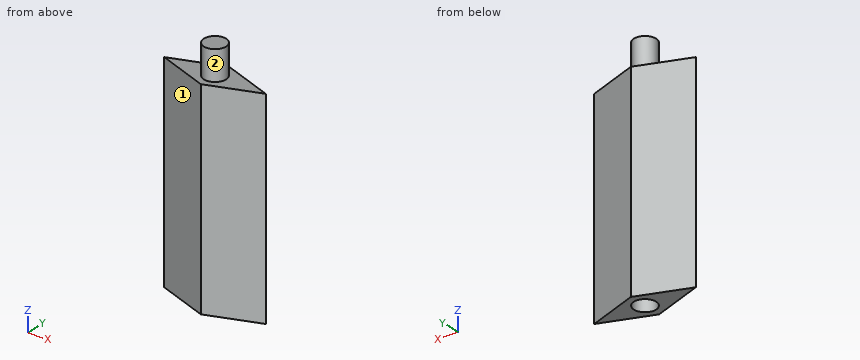
from build123d import *

# Parameters (mm, degrees)
F0_W        = 101.6
F0_H        = 31.75
F1_DEPTH    = 177.8
F2_T1_DEPTH = 441.3701848271
F3_R        = 9.525
F4_DEPTH    = 25.4
F5_R        = 9.525
F6_DEPTH    = 25.4


# Not quite as in the source:
# - a fillet or chamfer that OpenCascade refuses, or shapes differently, is made with other operations: its cross-section is extruded or revolved along the edge and cut away or added


with BuildPart() as f1:
    # F0 (on Top) → F1 (new body)
    with BuildSketch(Plane.XY):
        Rectangle(F0_W, F0_H)
    extrude(amount=F1_DEPTH)

    # F2: chamfer of 50.8 x 18.4896879007 on 4 edges, made by hand

    # F2_s2 → F2_t1 (cut)
    with BuildSketch(Plane.XY.offset(-131.7850924136)):
        Polygon((50.8, -2.6146879007), (0, 15.875), (50.8, 15.875), align=None)
        Polygon((50.8, 2.6146879007), (0, -15.875), (50.8, -15.875), align=None)
        Polygon((-50.8, 2.6146879007), (0, -15.875), (-50.8, -15.875), align=None)
        Polygon((0, 15.875), (-50.8, -2.6146879007), (-50.8, 15.875), align=None)
    extrude(amount=F2_T1_DEPTH, mode=Mode.SUBTRACT)

    # F3 (on face) → F4 (join)
    with BuildSketch(Plane.XY.offset(177.8)):
        Circle(F3_R)
    extrude(amount=F4_DEPTH)

    # F5 (on face) → F6 (cut)
    with BuildSketch(Plane(origin=(0, 0, 0), x_dir=(1, 0, 0), z_dir=(0, 0, -1))):
        Circle(F5_R)
    extrude(amount=-F6_DEPTH, mode=Mode.SUBTRACT)


solid = f1.part
Source: CAD feature listing. Evaluate the final solid. Frame: model axes, mm. Face numbers are marked on the shaded views. A direction names the side the tool comes from. Round coordinates to 2 decimals unless told otherwise and drop trailing zeros. Write each loop counter-clockwise with the first axis right and the second up, starting at its lowest first coordinate (ties: lowest second). Pieces come first, ordered by that corner, then holes. Notation, with made-up numbers: M 22.5,-33 L 31.5,-33 A5 ccw 31.5,-29 Z; hole C 71.5,70.25 d8. An arc over 180 degrees is marked long. One line per item, written item: value. Start each with the question number.
Item 1: Ray query, L1, parallel to Y at x = 0, z = 19 (3 decimals); L2, parallel to Z at x = 26.5, y = 6; L3, parallel to Y at x = -35, z = 125. Return the intervals inside material, ascending. Write a range as from..to.
Item 2: Section query B-B (y = 3.5). Return the cut outline in (x, z).
Item 3: Section query D-D (x = -21). Return the cut outline in (y, z).
Item 4: Section query C-C (z = 142.5). Return the cut outline in (x, y) (3 decimals).
Item 5: Set-up query: the marked faces 1 and 2. Return all of +Z, -Z, +X, -X, +Y, -Y with unobstructed straight access to the full face (end or side cutting, diameter ignored); none if empty.
Item 6: Pin query (flat end, axial travel): pin 1 (4 mm diameter, centred on x = 12, y = -11, fed in from +Z); pin 2 (15 mm diameter, centred on x = 0, y = 0, fed in from -Z); pin 3 (1 mm diameter, centred on y = 0, z = 84, fed in from +X). Return the tip coordinate at first contact, or that it passes through.
Item 7: Section query A-A (x = 6). Return the cut outline in (y, z).
Result set:
1. L1: y = -15.875..-9.525, 9.525..15.875
1. L2: z = 0..177.8
1. L3: y = -3.14..3.14
2. outline: M -34,0 L -8.86,0 L -8.86,25.4 L 8.86,25.4 L 8.86,0 L 34,0 L 34,177.8 L 8.86,177.8 L 8.86,203.2 L -8.86,203.2 L -8.86,177.8 L -34,177.8 Z
3. outline: M -8.23,0 L 8.23,0 L 8.23,177.8 L -8.23,177.8 Z
4. outline: M -43.616,0 L 0,-15.875 L 43.616,0 L 0,15.875 Z
5. face 1: +Z, -Z, -X, -Y
5. face 2: +Z
6. pin 1: stops at z = 177.8
6. pin 2: stops at z = 25.4
6. pin 3: stops at x = 43.62
7. outline: M -13.69,0 L -7.4,0 L -7.4,25.4 L 7.4,25.4 L 7.4,0 L 13.69,0 L 13.69,177.8 L 7.4,177.8 L 7.4,203.2 L -7.4,203.2 L -7.4,177.8 L -13.69,177.8 Z
